```python
from build123d import *

# Parameters (mm, degrees)
F0_R     = 6.35
F1_DEPTH = 30
F2_W     = 4
F2_H     = 16.105262
F3_DEPTH = 10


with BuildPart() as f1:
    # F0 (on Front) → F1 (new body)
    with BuildSketch(Plane.XZ):
        Circle(F0_R)
    extrude(amount=F1_DEPTH)

    # F2 (on face) → F3 (cut)
    with BuildSketch(Plane.XZ.offset(30)):
        Rectangle(F2_W, F2_H)
    extrude(amount=-F3_DEPTH, mode=Mode.SUBTRACT)


solid = f1.part
```
Input: part model. Units: mm. Frame: model coordinates. A direction names the side the tool comes from. Coordinates: 2 decimals unless noted, no trailing zeros. Loops run counter-clockwise (first coordinate to the right, second up) from the corner with the lowest first, then second, coordinate; pieces in that order, holes last. Notation, with made-up numbers: M -10,87.5 L 0,87.5 A14 ccw 0,105.5 Z; hole C 10,35.25 d10. An arc over 180 degrees is marked long. One line per item, written item: value.
(1) Pin query (flat end, axial travel): pin 1 (5 mm diameter, centred on y = -13.5, z = -3, fed in from +X); pin 2 (1.2 mm diameter, centred on x = -0.5, z = -3, fed in from -Y). Return the tip coordinate at first contact, or that it passes through.
Filled in:
pin 1: x = 6.33
pin 2: y = -20
(2) Line query: line 1 along Y through (x, z) = (-1.25, 1.75); line 2 along X through (y, z) = (-17, -2); line 3 along X through (y, z) = (-2.5, 0.25). Output: solid intervals per line, ascending. Write a range as from..to.
Filled in:
line 1: -20..0
line 2: -6.03..6.03
line 3: -6.35..6.35
(3) Reachability of faces 1 (the flat face through (2, -25, 0)), 2 (the flat face through (4, -30, 0)) from +Z, -Z, +X, -X, +Y, -Y: full face, straight path, thin tool, end or side. Return the list, or none.
Filled in:
face 1: +Z, -Z, -Y
face 2: +Z, -Z, +X, -X, -Y
(4) Section D-D (z = -4.5). Output: boundary loops of the cut face in (x, y).
Filled in:
outline: M -4.48,-30 L -2,-30 L -2,-20 L 2,-20 L 2,-30 L 4.48,-30 L 4.48,0 L -4.48,0 Z
(5) Section B-B (x = 0). Output: boundary loops of the cut face in (y, z), and give its area (3 significant figures).
Filled in:
outline: M -20,-6.35 L 0,-6.35 L 0,6.35 L -20,6.35 Z
area: 254 mm^2
(6) Section C-C (y = -12.25). Output: boundary loops of the cut face in (x, z), and give its area (3 significant figures).
Filled in:
outline: C 0,0 d12.7
area: 127 mm^2
(7) Section A-A (z = 0). Output: boundary loops of the cut face in (x, y).
Filled in:
outline: M -6.35,-30 L -2,-30 L -2,-20 L 2,-20 L 2,-30 L 6.35,-30 L 6.35,0 L -6.35,0 Z
(8) Pull-direction query (X, two-part tool) for faces 3 (the flat face through (0, 0, 0)), 4 (the cylindrical face through (6.057, -14.79, 1.907)), 5 (the flat face through (-2, -25, 0)); classes: +X half, -X half, draft (parallel to the pull), parting line (faces both ways), or undercut.
Filled in:
face 3: draft
face 4: parting line
face 5: undercut
